Read the model definition and answer for the solid it produces. Units are mm, in the model's axes. Face numbers are marked on the shaded views. A direction names the side the tool comes from. Give positions to 0.01 mm unless a question says otherwise; leave off trailing zeros. Write each loop counter-clockwise with the first axis right and the second up, starting at its lowest first coordinate (ties: lowest second). Pieces come first, ordered by that corner, then holes. Notation, with made-up numbers: (57.25, 6) -> (92.25, 6) arc R17 ccw to (92.25, 35) -> close; hole circle Ø9 at (35.25, -4.75). An arc over 180 degrees is marked (long way). Use a Markdown table: item, result.
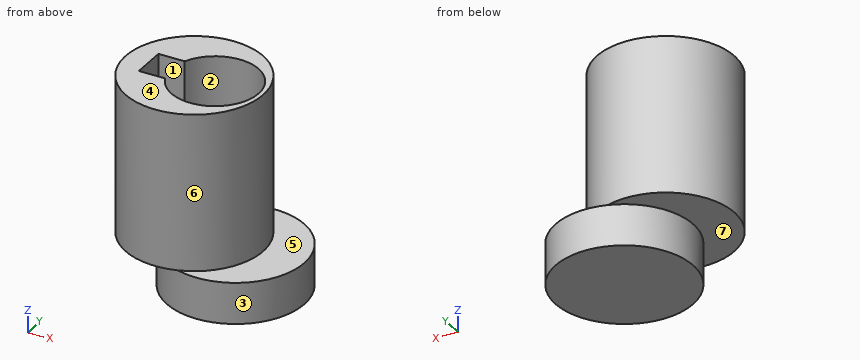
from build123d import *

# Parameters (mm, degrees)
SKETCH_1_R          = 10
EXTRUDE_1_DEPTH     = 6
SKETCH_2_R          = 10
EXTRUDE_2_DEPTH     = 22.8
CUT_EXTRUDE_1_DEPTH = 13


with BuildPart() as part:
    # 草图1 → 凸台-拉伸1 (new body)
    with BuildSketch(Plane.XY):
        Circle(SKETCH_1_R)
    extrude(amount=EXTRUDE_1_DEPTH)

    # 草图2 → 凸台-拉伸2 (add)
    with BuildSketch(Plane.XY.offset(6)):
        with Locations(Location((-6, 0, 0), (0, 0, 287.457603124))):
            Circle(SKETCH_2_R)
    extrude(amount=EXTRUDE_2_DEPTH)

    # 草图3 → 切除-拉伸1 (cut)
    with BuildSketch(Plane.XY.offset(28.8)):
        with BuildLine():
            Line((-12.65, 2.5), (-8.837165408, 2.5))
            ThreePointArc((-8.837165408, 2.5), (3.35, 0), (-8.837165408, -2.5))
            Line((-8.837165408, -2.5), (-12.65, -2.5))
            Line((-12.65, -2.5), (-12.65, 2.5))
        make_face()
    extrude(amount=-CUT_EXTRUDE_1_DEPTH, mode=Mode.SUBTRACT)


solid = part.part
Item 1: A cutting plane is placed at A-A (z = 21). Give the vertices of the cut face in (x, y), then the cut area to 3 significant figures.
Return value:
| item | result |
|---|---|
| outline | circle Ø20 at (-6, 0); hole (-12.65, -2.5) -> (-8.84, -2.5) arc R6.35 ccw (long way) to (-8.84, 2.5) -> (-12.65, 2.5) -> close |
| area | 170 mm^2 |
Item 2: A cutting plane is placed at C-C (y = -1). Give the vertices of the cut face in (x, z).
Return value:
| item | result |
|---|---|
| outline | (-15.95, 6) -> (-9.95, 6) -> (-9.95, 0) -> (9.95, 0) -> (9.95, 6) -> (3.95, 6) -> (3.95, 28.8) -> (3.27, 28.8) -> (3.27, 15.8) -> (-12.65, 15.8) -> (-12.65, 28.8) -> (-15.95, 28.8) -> close |
Item 3: Straight lines are drawn through the part: line 1 along X through (y, z) = (0, 24); line 2 along Z through (x, y) = (1, -2.25); line 3 along X through (y, z) = (-1.75, 24.5). For each, find the intervals that lie inside material, in ascending order. Write a range as [from, to].
Return value:
| item | result |
|---|---|
| line 1 | [-16, -12.65], [3.35, 4] |
| line 2 | [0, 15.8] |
| line 3 | [-15.85, -12.65], [3.1, 3.85] |
Item 4: Each of these flat-tipped pins is pushed along its axis until it touches: P1, Ø4, axis at x = -5.5, z = 17, coming from the +Y side; P2, Ø1.5, axis at y = 2, z = 19, coming from the +X side; P3, Ø1.5, axis at x = 0, z = 25, coming from the -Y side; P4, Ø1.5, axis at x = -11, z = 8, coming from the +Y side. Where does it stop, or does it pass through?
Return value:
| item | result |
|---|---|
| P1 | y = 10 |
| P2 | x = 3.92 |
| P3 | y = -8.51 |
| P4 | y = 9.05 |
Item 5: A cutting plane is placed at B-B (x = -6). Give the vertices of the cut face in (y, z), then the cut area to 3 significant figures.
Return value:
| item | result |
|---|---|
| outline | (-10, 6) -> (-8, 6) -> (-8, 0) -> (8, 0) -> (8, 6) -> (10, 6) -> (10, 28.8) -> (5.6, 28.8) -> (5.6, 15.8) -> (-5.6, 15.8) -> (-5.6, 28.8) -> (-10, 28.8) -> close |
| area | 406 mm^2 |
Item 6: A tool of negligible diameter and unlimited length cuts with its end or side. For the marked faces 5, 6 and 7, from which of +Z, -Z, +X, -X, +Y, -Y can it reach the whole face along a straight path? Write none if from no direction.
Return value:
| item | result |
|---|---|
| face 5 | +Z, +X |
| face 6 | +Z |
| face 7 | -Z, -X |
Item 7: For a pull along X with two mould halves and no side action, classify the marked faces 1, 2, 3 and 4 as +X half, -X half, draft (parallel to the pull), parting line (faces both ways), or undercut.
Return value:
| item | result |
|---|---|
| face 1 | undercut |
| face 2 | undercut |
| face 3 | parting line |
| face 4 | draft |
Item 8: A cutting plane is placed at D-D (z = 8.25). Give the vertices of the cut face in (x, y).
Return value:
| item | result |
|---|---|
| outline | circle Ø20 at (-6, 0) |
